Here's how the part is built. I have some questions about the finished solid (model axes, mm). A direction names the side the tool comes from. Coordinates: 2 decimals unless noted, no trailing zeros. Loops run counter-clockwise (first coordinate to the right, second up) from the corner with the lowest first, then second, coordinate; pieces in that order, holes last.
from build123d import *

# Parameters (mm, degrees)
F0_W      = 400
F0_H      = 150
F1_DEPTH  = 12
F2_W      = 12
F2_H      = 150
F3_DEPTH  = 200
F4_W      = 12
F4_H      = 150
F5_DEPTH  = 200
F6_W      = 400
F6_H      = 150
F7_DEPTH  = 12
F9_D      = 80
F9_DEPTH  = 12
F10_D     = 80
F10_DEPTH = 12
F11_D     = 80
F11_DEPTH = 12


with BuildPart() as f1:
    # F0 (on Top) → F1 (new body)
    with BuildSketch(Plane.XY):
        with Locations((200, 75)):
            Rectangle(F0_W, F0_H)
    extrude(amount=F1_DEPTH)

    # F2 (on face) → F3 (join)
    with BuildSketch(Plane.XY.offset(12)):
        with Locations((6, 75)):
            Rectangle(F2_W, F2_H)
    extrude(amount=F3_DEPTH)

    # F4 (on face) → F5 (join)
    with BuildSketch(Plane.XY.offset(12)):
        with Locations((394, 75)):
            Rectangle(F4_W, F4_H)
    extrude(amount=F5_DEPTH)

    # F6 (on face) → F7 (join)
    with BuildSketch(Plane.XY.offset(212)):
        with Locations((200, 75)):
            Rectangle(F6_W, F6_H)
    extrude(amount=F7_DEPTH)

    # F9
    with Locations(Plane.XY.offset(224)):
        with Locations((80, 75)):
            Hole(F9_D / 2, depth=F9_DEPTH)

    # F10
    with Locations(Plane.XY.offset(224)):
        with Locations((200, 75)):
            Hole(F10_D / 2, depth=F10_DEPTH)

    # F11
    with Locations(Plane.XY.offset(224)):
        with Locations((320, 75)):
            Hole(F11_D / 2, depth=F11_DEPTH)


solid = f1.part
Q1. For faces 1 (the cylindrical face through (41.847, 87.015, 217.916)), 2 (the flat face through (197, 76, 12)), 3 (the flat face through (0, 74, 110)), which set-ups out of +Z, -Z, +X, -X, +Y, -Y let a thin tool reach every point of the face, with its end or its side?
Q2. We'd pull the mould along Z, two halves only. Please class faces 4 (the flat face through (12, 74, 111)), 5 (the cylindrical face through (359.96, 76.76, 217.92)), 6 (the flat face through (153, 76, 224)), 7 (the flat face through (197, 76, 0)): pulls with the +Z half, pulls with the -Z half, needs draft (parallel to the pull), parting line crosses it, or undercut.
Q3. Suppose I cut it at A-A on z = 204.5. Write out the boundary of the cut face in (x, y).
Q4. Suppose I cut it at D-D on y = 125. Write out the boundary of the cut face in (x, z), and give its area (3 significant figures).
Q5. Will this pin go through, and if not, where does the flat tip stop? P1, Ø8, axis at x = 299, y = 59, coming from the +Z side.
Q6. Suppose I cut it at C-C on x = 320. Write out the boundary of the cut face in (y, z), and give its area (3 significant figures).
Q7. Suppose I cut it at B-B on x = 144.5. Write out the boundary of the cut face in (y, z), and give its area (3 significant figures).
Q8. Please list where these lines run through material, in increasing order: probe 1 along X at (y, z) = (114, 47); probe 2 along Y at (x, z) = (320, 219); probe 3 along Z at (x, y) = (56, 24.5).
Check values:
1. face 1: +Z
1. face 2: +Y, -Y
1. face 3: +Z, -Z, -X, +Y, -Y
2. face 4: undercut
2. face 5: needs draft
2. face 6: pulls with the +Z half
2. face 7: pulls with the -Z half
3. outline: (0, 0) - (12, 0) - (12, 150) - (0, 150) - close; (388, 0) - (400, 0) - (400, 150) - (388, 150) - close
4. outline: (0, 0) - (400, 0) - (400, 224) - (0, 224) - close; hole (12, 12) - (388, 12) - (388, 212) - (12, 212) - close
4. area: 14,400 mm2
5. P1: stops at z = 12
6. outline: (0, 0) - (150, 0) - (150, 12) - (0, 12) - close; (0, 212) - (35, 212) - (35, 224) - (0, 224) - close; (115, 212) - (150, 212) - (150, 224) - (115, 224) - close
6. area: 2,640 mm2
7. outline: (0, 0) - (150, 0) - (150, 12) - (0, 12) - close; (0, 212) - (150, 212) - (150, 224) - (0, 224) - close
7. area: 3,600 mm2
8. probe 1: x = 0 to 12, 388 to 400
8. probe 2: y = 0 to 35, 115 to 150
8. probe 3: z = 0 to 12, 212 to 224
